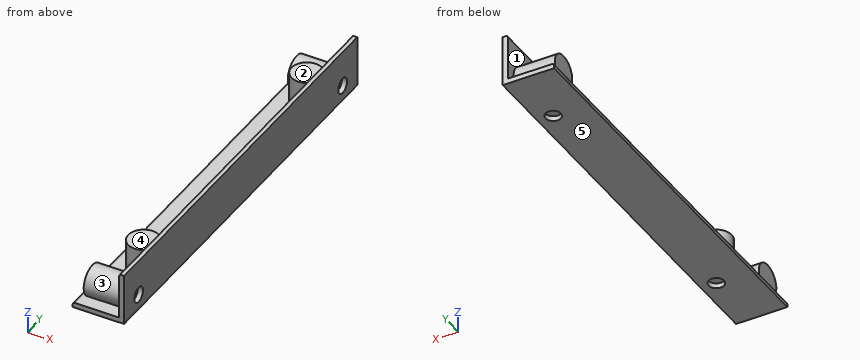
from build123d import *

# Parameters (mm, degrees)
F1_DEPTH = 400
F2_R     = 7.5
F3_DEPTH = 5
F4_R     = 7.5
F5_DEPTH = 5
F6_R     = 15
F7_DEPTH = 40
F8_R     = 15
F9_DEPTH = 40


with BuildPart() as f1:
    # F0 (on Front) → F1 (new body)
    with BuildSketch(Plane.XZ):
        with BuildLine():
            Line((0, 50), (-3, 50))
            ThreePointArc((-3, 50), (-4.414214, 49.414214), (-5, 48))
            Line((-5, 48), (-5, 5))
            Line((-5, 5), (-48, 5))
            ThreePointArc((-48, 5), (-49.414214, 4.414214), (-50, 3))
            Line((-50, 3), (-50, 0))
            Line((-50, 0), (0, 0))
            Line((0, 0), (0, 50))
        make_face()
    extrude(amount=F1_DEPTH)

    # F2 (on face) → F3 (cut, through all)
    with BuildSketch(Plane(origin=(-5, 0, 0), x_dir=(0, -1, 0), z_dir=(-1, 0, 0))):
        with Locations((25, 15)):
            Circle(F2_R)
        with Locations((375, 15)):
            Circle(F2_R)
    extrude(amount=-F3_DEPTH, mode=Mode.SUBTRACT)

    # F4 (on face) → F5 (cut, through all)
    with BuildSketch(Plane.XY.offset(5)):
        with Locations((-15, -60)):
            Circle(F4_R)
        with Locations((-15, -340)):
            Circle(F4_R)
    extrude(amount=-F5_DEPTH, mode=Mode.SUBTRACT)

    # F6 (on face) → F7 (join)
    with BuildSketch(Plane(origin=(-5, 0, 0), x_dir=(0, -1, 0), z_dir=(-1, 0, 0))):
        with Locations((375, 15)):
            Circle(F6_R)
        with Locations((25, 15)):
            Circle(F6_R)
    extrude(amount=F7_DEPTH)

    # F8 (on face) → F9 (join)
    with BuildSketch(Plane.XY.offset(5)):
        with Locations((-15, -340)):
            Circle(F8_R)
        with Locations((-15, -60)):
            Circle(F8_R)
    extrude(amount=F9_DEPTH)


solid = f1.part
Check sheet for the modelled part. Datum: model origin and axes. Units: mm. Face numbers are marked on the shaded views. A direction names the side the tool comes from. Give positions to 0.01 mm unless a question says otherwise; leave off trailing zeros. Write each loop counter-clockwise with the first axis right and the second up, starting at its lowest first coordinate (ties: lowest second). Pieces come first, ordered by that corner, then holes. Notation, with made-up numbers: (55, 76) -> (107, 76) arc R17 cw to (107, 93) -> close; hole circle Ø11 at (51, 18.5). An arc over 180 degrees is marked (long way). Use one line per item in the form item = value. Start each with the question number.
1. Go/stop test with flat-tipped pins: P1, Ø13, axis at y = -174.5, z = 34, coming from the -X side; P2, Ø12, axis at y = -350.5, z = 39, coming from the -X side; P3, Ø4.5, axis at x = -17.5, y = -339, coming from the -Z side. Record where each tip stops, or that it passes through.
2. Thickness scan on line 1 along Y through (x, z) = (-15, 1); line 2 along X through (y, z) = (-340, 2.8); line 3 along Y through (x, z) = (-16, 37). Record the ranges inside material, lowest first. Write a range as from..to.
3. Section check B-B (z = 15). Record the cut outline in (x, y), and give its area (3 significant figures).
4. Section check D-D (y = -169). Record the cut outline in (x, z).
5. Section check C-C (x = -18.5). Record the cut outline in (y, z), and give its area (3 significant figures).
6. Mould release check, pull along Y, two halves, no side actions. Record for the marked faces 1, 2 and 3: pulls with the +Y half, pulls with the -Y half, needs draft (parallel to the pull), parting line crosses it, or undercut.
7. Access from +Z, -Z, +X, -X, +Y, -Y to the whole of each face (thin tool, end or side, straight path). Record for the marked faces 4 and 5.
8. Section check A-A (y = -25). Record the cut outline in (x, z), and give its area (3 significant figures).
Conclusion:
q1.P1 = -5
q1.P2 = -29.31
q1.P3 = 5
q2.line_1 = -400..-347.5, -332.5..-67.5, -52.5..0
q2.line_2 = -50..-22.5, -7.5..0
q2.line_3 = -354.97..-325.03, -74.97..-45.03
q3.outline = (-45, -390) -> (-5, -390) -> (-5, -400) -> (0, -400) -> (0, -382.5) -> (-5, -382.5) -> (-5, -367.5) -> (0, -367.5) -> (0, -32.5) -> (-5, -32.5) -> (-5, -17.5) -> (0, -17.5) -> (0, 0) -> (-5, 0) -> (-5, -10) -> (-45, -10) -> (-45, -40) -> (-5, -40) -> (-5, -48.82) arc R15 ccw (long way) to (-5, -71.18) -> (-5, -328.82) arc R15 ccw (long way) to (-5, -351.18) -> (-5, -360) -> (-45, -360) -> close
q3.area = 5,510 mm²
q4.outline = (-50, 0) -> (0, 0) -> (0, 50) -> (-3, 50) arc R2 ccw to (-5, 48) -> (-5, 5) -> (-48, 5) arc R2 ccw to (-50, 3) -> close
q5.outline = (-400, 0) -> (-346.63, 0) -> (-346.63, 5) -> (-333.37, 5) -> (-333.37, 0) -> (-66.63, 0) -> (-66.63, 5) -> (-53.37, 5) -> (-53.37, 0) -> (0, 0) -> (0, 5) -> (-13.82, 5) arc R15 ccw (long way) to (-36.18, 5) -> (-45.41, 5) -> (-45.41, 45) -> (-74.59, 45) -> (-74.59, 5) -> (-325.41, 5) -> (-325.41, 45) -> (-354.59, 45) -> (-354.59, 5) -> (-363.82, 5) arc R15 ccw (long way) to (-386.18, 5) -> (-400, 5) -> close
q5.area = 5,460 mm²
q6.face_1 = undercut
q6.face_2 = needs draft
q6.face_3 = undercut
q7.face_4 = +Z, -X, +Y, -Y
q7.face_5 = -Z, +X, -X, +Y, -Y
q8.outline = (-50, 0) -> (0, 0) -> (0, 7.5) -> (-5, 7.5) -> (-5, 22.5) -> (0, 22.5) -> (0, 50) -> (-3, 50) arc R2 ccw to (-5, 48) -> (-5, 30) -> (-45, 30) -> (-45, 5) -> (-48, 5) arc R2 ccw to (-50, 3) -> close
q8.area = 1,400 mm²
